Autodesk Inventor part; units mm, degrees
ref_plane "YZ Plane" through (0, 0, 0) normal (1, 0, 0) x (0, 1, 0)
ref_plane "XZ Plane" through (0, 0, 0) normal (0, 1, 0) x (-1, 0, 0)
ref_plane "XY Plane" through (0, 0, 0) normal (0, 0, 1) x (1, 0, 0)
sketch "Sketch1" plane through (0, 0, 0) normal (0, 0, 1) x (1, 0, 0)
  line L0 (1.4434, 2.5) -> (2.8868, 0)
  line L1 (2.8868, 0) -> (1.4434, -2.5)
  line L2 (1.4434, -2.5) -> (-1.4434, -2.5)
  line L3 (-1.4434, -2.5) -> (-2.8868, 0)
  line L4 (-2.8868, 0) -> (-1.4434, 2.5)
  line L5 (-1.4434, 2.5) -> (1.4434, 2.5)
  point P0 (0, 0)
  point P1 (0, 0)
  dimension "d0" = 5
extrude "Extrusion1" add sketch "Sketch1" along normal blind 10
sketch "Sketch3" plane through (0, 0, 0) normal (0, 0, -1) x (-1, 0, 0)
  line L0 (1.4434, 2.5) -> (-1.4434, 2.5)
  circle A0 centre (0, 0) radius 2.5
hole "Hole1" at (0, 0, 0) direction (0, 0, 1) diameter 2.459 end through all
chamfer "Chamfer2" distance 0.5 angle 45 1 edges at (0, -1.2295, 0)
sketch "Sketch4" plane through (0, 0, 0) normal (0, 0, -1) x (-1, 0, 0)
  circle A0 centre (0, 0) radius 1.7295
  circle A1 centre (0, 0) radius 2.5
  circle A2 centre (0, 0) radius 6
extrude "Extrusion3" cut sketch "Sketch4" against normal blind 1 draft -45 contours A2
ref_plane "Work Plane1" through (0, 0, 5) normal (0, 0, -1) x (-1, 0, 0)
mirror "Mirror2" about plane through (0, 0, 5) normal (0, 0, -1) of "Extrusion3"
chamfer "Chamfer3" distance 0.5 angle 45 1 edges at (0, -1.2295, 10)
properties part number "support m3 10" material "Stainless Steel"
Can you work these out from the model? Positions are in its coordinate system, mm. Give positions to 0.01 mm unless a question says otherwise; leave off trailing zeros. Order: outer loops, then holes, each group sorted by start corner. A loop starts at its lowest first (then second) coordinate and runs counter-clockwise, first axis right, second up. Notation, with made-up numbers: (-17, 7) - (-4, 7) arc R19 ccw to (-4, 24) - close; hole circle Ø9 at (0, 2.25). An arc over 180 degrees is marked (long way). Use a Markdown table: item, result. Add a question column.
Q1. If we section it at A-A on z = 1.75: Write out the boundary of the cut face in (x, y).
Q2. I'm going to push flat-ended pins straight in: pin 1 (3 mm diameter, centred on x = 0, y = 0, fed in from +Z); pin 2 (1.5 mm diameter, centred on y = -1, z = 4.5, fed in from -X). Where does each tip first touch, or does it pass through?
Q3. If we mould it in two halves opening along X, with no side actions, what happens to faces 1 (the cylindrical face through (0.748, -0.976, 5.063)), 2 (the conical face through (1.317, 2.268, 0.123)), 3 (the flat face through (2, 1, 10))? For each: released by +X, released by -X, zero draft, split by the parting line, or undercut.
Q4. Please list where these lines run through material, in increasing order: line 1 along Y through (x, z) = (0, 6); line 2 along X through (y, z) = (-0.9, 2.5); line 3 along X through (y, z) = (1.05, 1).
Answers follow:
| question | item | result |
|---|---|---|
| 1 | outline | (-2.89, 0) - (-1.44, -2.5) - (1.44, -2.5) - (2.89, 0) - (1.44, 2.5) - (-1.44, 2.5) - close; hole circle Ø2.46 at (0, 0) |
| 2 | pin 1 | stops at z = 9.77 |
| 2 | pin 2 | stops at x = -2.74 |
| 3 | face 1 | undercut |
| 3 | face 2 | released by +X |
| 3 | face 3 | zero draft |
| 4 | line 1 | y = -2.5 to -1.23, 1.23 to 2.5 |
| 4 | line 2 | x = -2.37 to -0.84, 0.84 to 2.37 |
| 4 | line 3 | x = -2.28 to -0.64, 0.64 to 2.28 |
